The figure shows three views and two pictorial views of one solid part (mm, origin at its lowest corner). Answer the questions. Coordinates: 2 decimals unless noted, no trailing zeros. Loops run counter-clockwise (first coordinate to the right, second up) from the corner with the lowest first, then second, coordinate; pieces in that order, holes last. Notation, with made-up numbers: (-31.5, -20.75) - (15.5, -20.75) arc R22 ccw to (15.5, 11.25) - close; hole circle Ø10 at (-33.75, -20). An arc over 180 degrees is marked (long way). Write each question's results on one line, items separated by ' | '. Start each with the question number.
Item 1: Section D-D, the plane z = 18 is taken. Write down the section's boundary in (x, y).
Item 2: For a pull along Z with two mould halves and no side action, classify the marked faces 1, 2 and 3 as +Z half, -Z half, draft (parallel to the pull), parting line (faces both ways), or undercut.
Item 3: Each of these flat-tipped pins is pushed along its axis until it touches: pin 1 Ø6 at (x, z) = (7.5, 14) entering from +Y; pin 2 Ø6 at (x, y) = (4, 16) entering from +Z; pin 3 Ø1.5 at (x, z) = (4, 6.5) entering from +Y. Where does it stop, or does it pass through?
Item 4: Section C-C, the plane x = 1.5 is taken. Write down the section's boundary in (y, z), plus the area to 3 significant figures.
Item 5: Consider probe 1 along Y at (x, z) = (7.75, 10); probe 2 along Z at (x, y) = (5.5, 2); probe 3 along Z at (x, y) = (7.75, 9). Determine where each line is inside the solid, lowest interval first. Write a range as [from, to].
Item 6: Section A-A, the plane z = 10 is taken. Write down the section's boundary in (x, y), plus the area to 3 significant figures.
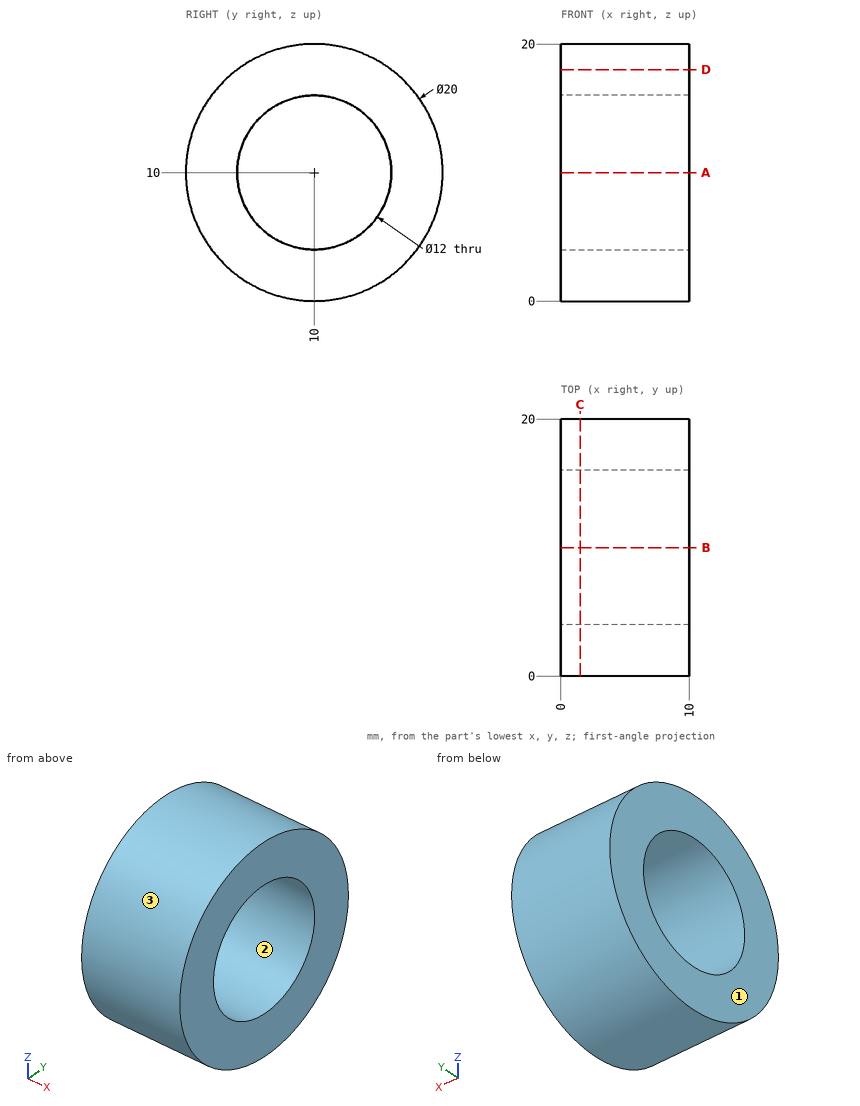
Answer key:
1) outline: (0, 4) - (10, 4) - (10, 16) - (0, 16) - close
2) face 1: draft | face 2: undercut | face 3: parting line
3) pin 1: stops at y = 19.95 | pin 2: stops at z = 19.54 | pin 3: stops at y = 19.61
4) outline: circle Ø20 at (10, 10); hole circle Ø12 at (10, 10) | area: 201 mm^2
5) probe 1: y = [0, 4], [16, 20] | probe 2: z = [4, 16] | probe 3: z = [0.05, 4.08], [15.92, 19.95]
6) outline: (0, 0) - (10, 0) - (10, 4) - (0, 4) - close; (0, 16) - (10, 16) - (10, 20) - (0, 20) - close | area: 80.0 mm^2
